```python
from build123d import *

# Parameters (mm, degrees)
BOSS_EXTRU_1_DEPTH = 10
D_GAGEMENT_M41_D   = 19


with BuildPart() as part:
    # Esquisse1 → Boss.-Extru.1 (new body)
    with BuildSketch(Plane.XY):
        with BuildLine():
            Line((0, 0), (0, 37.161178186))
            ThreePointArc((0, 37.161178186), (1.574901575, 54.838847716), (6.25, 71.959705454))
            ThreePointArc((6.25, 71.959705454), (13.580589093, 81.419410907), (25, 85))
            Line((25, 85), (55, 85))
            ThreePointArc((55, 85), (66.419410907, 81.419410907), (73.75, 71.959705454))
            ThreePointArc((73.75, 71.959705454), (78.425098425, 54.838847716), (80, 37.161178186))
            Line((80, 37.161178186), (80, 0))
            Line((80, 0), (0, 0))
        make_face()
    extrude(amount=BOSS_EXTRU_1_DEPTH)

    # Dégagement M41 (through all)
    with Locations(Plane.XY.offset(10)):
        with Locations((40, 64)):
            Hole(D_GAGEMENT_M41_D / 2)


solid = part.part
```
The model under review builds one solid part; all positions refer to its coordinate system, in mm. Give positions to 0.01 mm unless a question says otherwise; leave off trailing zeros. Write each loop counter-clockwise with the first axis right and the second up, starting at its lowest first coordinate (ties: lowest second). Pieces come first, ordered by that corner, then holes. Notation, with made-up numbers: (13, 27) -> (33, 27) arc R23 ccw to (33, 51) -> close; hole circle Ø10 at (43, 55.25). An arc over 180 degrees is marked (long way). Answer in a Markdown table with one row per item.
1) For L1, parallel to Y at x = 40, z = 7.5; L2, parallel to X at y = 38.5, z = 1.25; L3, parallel to Y at x = 47, z = 0.5, list the stretches that pass through material, from the lowest coordinate up. Write a range as [from, to].
Worked answers:
| item | result |
|---|---|
| L1 | [0, 54.5], [73.5, 85] |
| L2 | [0.01, 79.99] |
| L3 | [0, 57.58], [70.42, 85] |
2) Add section C-C on y = 64. State the section outline as (x, z) points, plus the area to 3 significant figures.
Worked answers:
| item | result |
|---|---|
| outline | (3.67, 0) -> (30.5, 0) -> (30.5, 10) -> (3.67, 10) -> close; (49.5, 0) -> (76.33, 0) -> (76.33, 10) -> (49.5, 10) -> close |
| area | 537 mm² |
3) Add section A-A on x = 40. State the section outline as (y, z) points, plus the area to 3 significant figures.
Worked answers:
| item | result |
|---|---|
| outline | (0, 0) -> (54.5, 0) -> (54.5, 10) -> (0, 10) -> close; (73.5, 0) -> (85, 0) -> (85, 10) -> (73.5, 10) -> close |
| area | 660 mm² |
4) Clearance check with a flat-ended pin moving along its axis: P1, Ø6, axis at x = 59, z = 1.5, coming from the +Y side (3 decimals). State where the tip first meets the part, or that it passes through.
Worked answers:
| item | result |
|---|---|
| P1 | y = 84.975 |
5) Add section B-B on z = 2. State the section outline as (x, y) points.
Worked answers:
| item | result |
|---|---|
| outline | (0, 0) -> (80, 0) -> (80, 37.16) arc R100 ccw to (73.75, 71.96) arc R20 ccw to (55, 85) -> (25, 85) arc R20 ccw to (6.25, 71.96) arc R100 ccw to (0, 37.16) -> close; hole circle Ø19 at (40, 64) |
6) Mouldability with a two-part tool opening along X and no side actions: class faces 1 (the cylindrical face through (1.53, 54.59, 4.93)), 2 (the cylindrical face through (34.89, 72.01, 4.93)), 3 (the cylindrical face through (78.38, 55.08, 4.93)), 4 (the flat face through (41, 43, 0)) as +X half, -X half, draft (parallel to the pull), parting line (faces both ways), or undercut.
Worked answers:
| item | result |
|---|---|
| face 1 | -X half |
| face 2 | undercut |
| face 3 | +X half |
| face 4 | draft |
